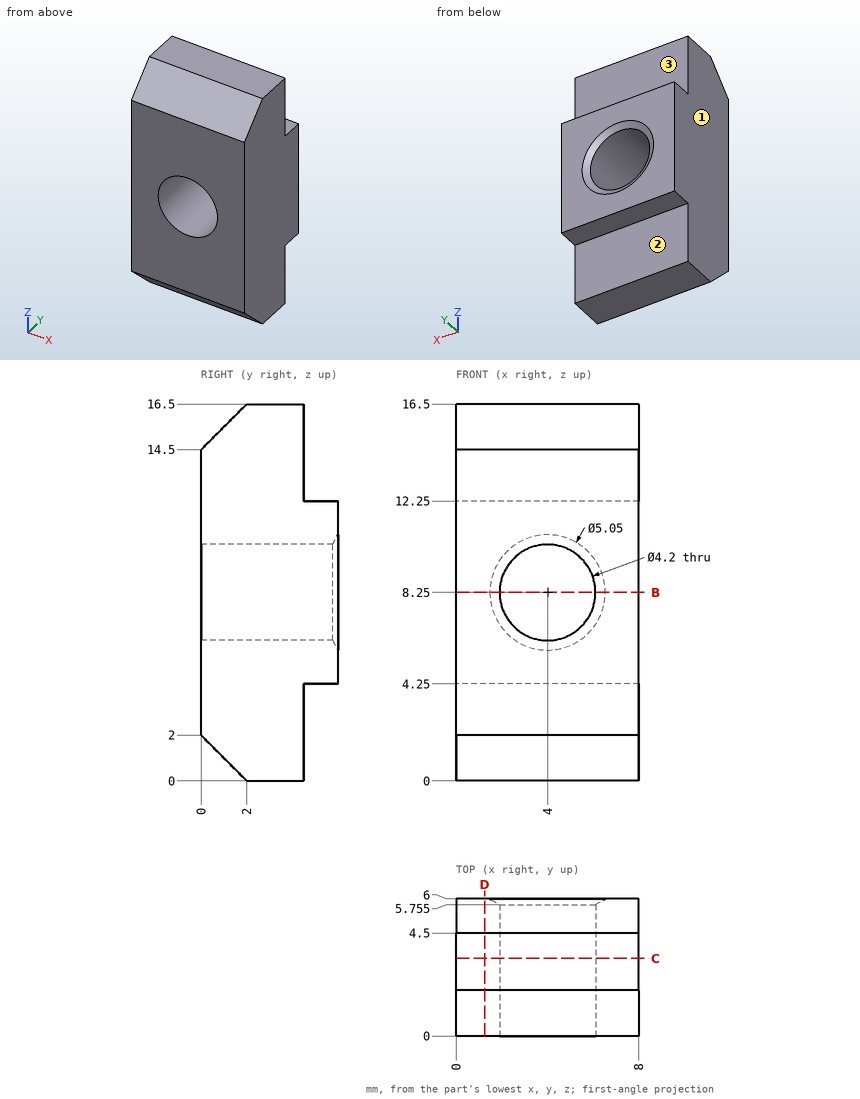
Source: three-view drawing plus pictorial views. Frame: mm from the lowest corner of the part. A direction names the side the tool comes from. Coordinates: 2 decimals unless noted, no trailing zeros. Order: outer loops, then holes, each group sorted by start corner. A loop starts at its lowest first (then second) coordinate and runs counter-clockwise, first axis right, second up. Notation, with made-up numbers: M 52.5,79 L 89.5,79 A16 cw 89.5,107 Z; hole C -38,-17.5 d4. An arc over 180 degrees is marked long. Write each question's results on one line, items separated by ' | '. Start each with the question number.
1. Pin query (flat end, axial travel): pin 1 (2 mm diameter, centred on x = 4.5, z = 15, fed in from +Y). Return the tip coordinate at first contact, or that it passes through.
2. Section B-B, the plane z = 8.25. Return the cut outline in (x, y) (1 decimal), then the cut area to 3 significant figures.
3. Reachability of the marked faces 1, 2 and 3 from +Z, -Z, +X, -X, +Y, -Y: full face, straight path, thin tool, end or side. Return the list, or none.
4. Section C-C, the plane y = 3.4. Return the cut outline in (x, z).
5. Section D-D, the plane x = 1.25. Return the cut outline in (y, z).
6. Material intervals for L1, parallel to Z at x = 4, y = 3.85; L2, parallel to Y at x = 6.75, z = 14.25; L3, parallel to Z at x = 0.75, y = 4.7, sorted ascending.
Solution:
1) pin 1: y = 4.5
2) outline: M 0,0 L 1.9,0 L 1.9,5.8 L 1.5,6 L 0,6 Z; M 6.1,0 L 8,0 L 8,6 L 6.5,6 L 6.1,5.8 Z | area: 22.7 mm²
3) face 1: +Z, -Z, -X, +Y, -Y | face 2: -Z, +X, -X, +Y | face 3: +Z, +X, -X, +Y
4) outline: M 0,0 L 8,0 L 8,16.5 L 0,16.5 Z; hole C 4,8.25 d4.2
5) outline: M 0,2 L 2,0 L 4.5,0 L 4.5,4.25 L 6,4.25 L 6,12.25 L 4.5,12.25 L 4.5,16.5 L 2,16.5 L 0,14.5 Z
6) L1: 0 to 6.15, 10.35 to 16.5 | L2: 0 to 4.5 | L3: 4.25 to 12.25
